CAD build for the part. Positions are in the model's coordinates, mm. Face numbers are marked on the shaded views. A direction names the side the tool comes from. Round coordinates to 2 decimals unless told otherwise and drop trailing zeros. Order: outer loops, then holes, each group sorted by start corner. A loop starts at its lowest first (then second) coordinate and runs counter-clockwise, first axis right, second up. Notation, with made-up numbers: M -25,76 L 19,76 A18 ccw 19,98 Z; hole C 1.5,-28 d5. An arc over 180 degrees is marked long. Answer as a JSON object with one key per item and string values. Group by question number.
```python
from build123d import *

# Parameters (mm, degrees)
F1_DEPTH = 1
F0_W     = 24
F0_H     = 2
F2_DEPTH = 3


with BuildPart() as f1:
    # F0 (on Top) → F1 (new body)
    with BuildSketch(Plane.XY):
        with BuildLine():
            Line((-12, 0), (12, 0))
            Line((12, 0), (4, 24))
            Line((4, 24), (4, 18.25))
            ThreePointArc((4, 18.25), (3.535534, 16.379171), (2.25, 14.942811))
            Line((2.25, 14.942811), (2.25, 12))
            ThreePointArc((2.25, 12), (0, 9.75), (-2.25, 12))
            Line((-2.25, 12), (-2.25, 14.942811))
            ThreePointArc((-2.25, 14.942811), (-3.535534, 16.379171), (-4, 18.25))
            Line((-4, 18.25), (-4, 24))
            Line((-4, 24), (-12, 0))
        make_face()
    extrude(amount=F1_DEPTH)

    # F0 (on Top) → F2 (join)
    with BuildSketch(Plane.XY):
        with Locations((0, -1)):
            Rectangle(F0_W, F0_H)
    extrude(amount=F2_DEPTH)


solid = f1.part
```
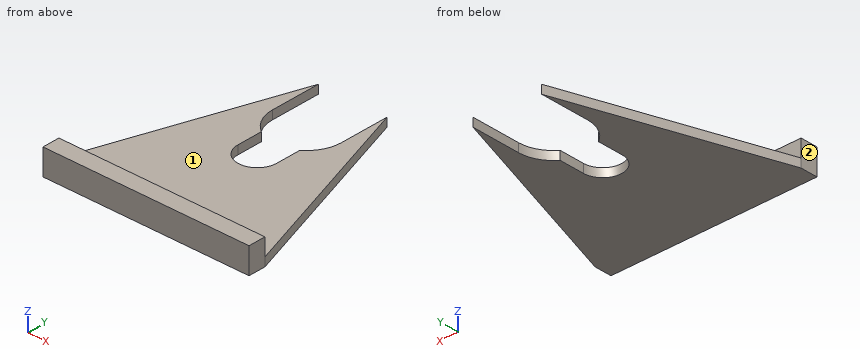
Item 1: Drill centre lines: line 1 (Y direction, x = 5.25, z = 2.6); line 2 (Z direction, x = -7.5, y = 0.5); line 3 (X direction, y = 14, z = 0.65). Where is each one in solid material? Low to high. Write a range as [from, to].
Item 2: 3-axis set-ups, long thin cutter, end or side, ignore diameter. For the marked faces 1 and 2: which of +Z, -Z, +X, -X, +Y, -Y reach the whole face in a straight line?
Item 3: Cut at A-A, the plane y = 13.5. Give the cut face in (x, z).
Item 4: Flat gauge pins, fed straight in: pin 1 Ø1 at (y, z) = (16.5, 2) entering from +X; pin 2 Ø6 at (x, y) = (4, 12) entering from -Z; pin 3 Ø7 at (x, y) = (0, 6) entering from +Z; pin 4 Ø1.1 at (y, z) = (13.5, 0.5) entering from +X. Where does each tip first touch, or does it go through?
Item 5: Cut at B-B, the plane x = 6.25. Give the cut face in (y, z).
Item 6: Cut at C-C, the plane y = 19. Give the cut face in (x, z), and give its area (3 significant figures).
Item 7: Cut at D-D, the plane z = 1.85. Give the cut face in (x, y), and give its area (3 significant figures).
Response values:
{
 "1": {"line 1": "[-2, 0]", "line 2": "[0, 1]", "line 3": "[-7.33, -2.25], [2.25, 7.33]"},
 "2": {"face 1": "+Z, +X, -X, +Y", "face 2": "+Z, -Z, -X, +Y, -Y"},
 "3": {"outline": "M -7.5,0 L -2.25,0 L -2.25,1 L -7.5,1 Z; M 2.25,0 L 7.5,0 L 7.5,1 L 2.25,1 Z"},
 "4": {"pin 1": "through", "pin 2": "z = 0", "pin 3": "z = 1", "pin 4": "x = 7.68"},
 "5": {"outline": "M -2,0 L 17.25,0 L 17.25,1 L 0,1 L 0,3 L -2,3 Z"},
 "6": {"outline": "M -5.67,0 L -4,0 L -4,1 L -5.67,1 Z; M 4,0 L 5.67,0 L 5.67,1 L 4,1 Z", "area": "3.33 mm^2"},
 "7": {"outline": "M -12,-2 L 12,-2 L 12,0 L -12,0 Z", "area": "48.0 mm^2"}
}
